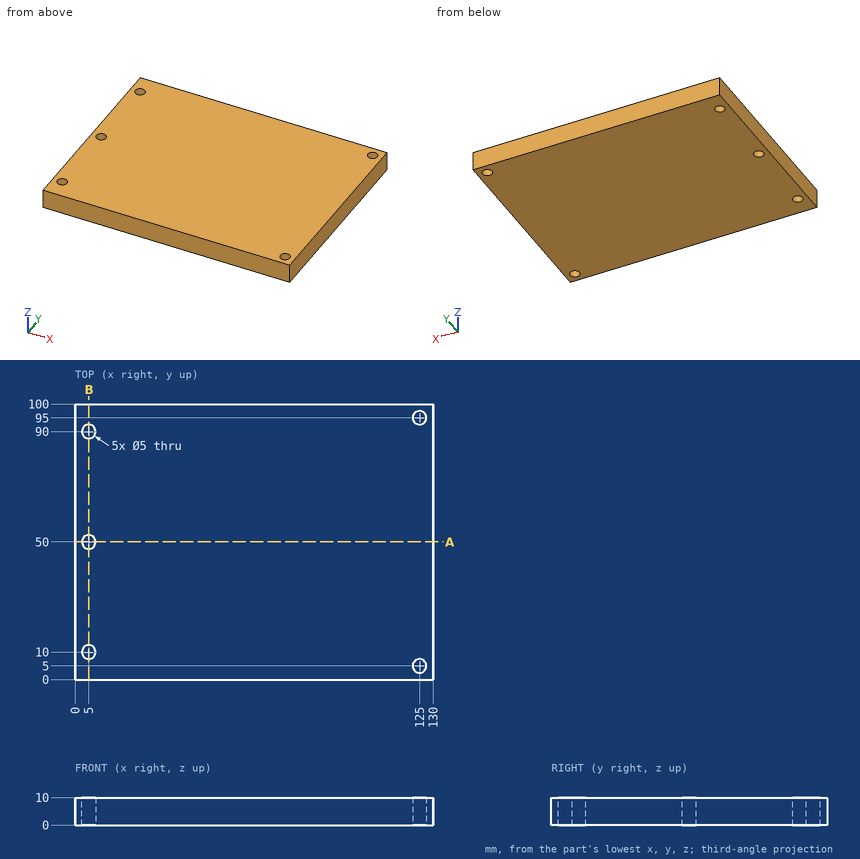
Here's the drawing with two shaded views (mm, measured from the low corner). I have some questions. Round coordinates to 2 decimals unless told otherwise and drop trailing zeros. Loops run counter-clockwise (first coordinate to the right, second up) from the corner with the lowest first, then second, coordinate; pieces in that order, holes last.
Item 1: Suppose I cut it at A-A, the plane y = 50. Write out the boundary of the cut face in (x, z), then the cut area to 3 significant figures.
Item 2: Please list where these lines run through material, in increasing order: L1, parallel to Y at x = 5, z = 3.25; L2, parallel to Y at x = 125, z = 4; L3, parallel to X at y = 90, z = 7.5.
Item 3: Suppose I cut it at B-B, the plane x = 5. Write out the boundary of the cut face in (y, z).
Item 4: Will this pin go through, and if not, where does the flat tip stop? pin 1 Ø3 at (x, y) = (125, 95) entering from +Z.
Reported:
1. outline: (0, 0) - (2.5, 0) - (2.5, 10) - (0, 10) - close; (7.5, 0) - (130, 0) - (130, 10) - (7.5, 10) - close
1. area: 1,250 mm2
2. L1: y = 0 to 7.5, 12.5 to 47.5, 52.5 to 87.5, 92.5 to 100
2. L2: y = 0 to 2.5, 7.5 to 92.5, 97.5 to 100
2. L3: x = 0 to 2.5, 7.5 to 130
3. outline: (0, 0) - (7.5, 0) - (7.5, 10) - (0, 10) - close; (12.5, 0) - (47.5, 0) - (47.5, 10) - (12.5, 10) - close; (52.5, 0) - (87.5, 0) - (87.5, 10) - (52.5, 10) - close; (92.5, 0) - (100, 0) - (100, 10) - (92.5, 10) - close
4. pin 1: passes through
